Autodesk Inventor part; units mm, degrees
ref_plane "YZ Plane" through (0, 0, 0) normal (1, 0, 0) x (0, 1, 0)
ref_plane "XZ Plane" through (0, 0, 0) normal (0, 1, 0) x (-1, 0, 0)
ref_plane "XY Plane" through (0, 0, 0) normal (0, 0, 1) x (1, 0, 0)
sketch "草圖1" plane through (0, 0, 0) normal (0, 0, 1) x (1, 0, 0)
  line L0 (0, 0) -> (0, 10) construction
  line L1 (1.25, 0) -> (1.25, 10)
  line L2 (-1.25, 10) -> (-1.25, 0)
  arc A0 (-1.25, 0) -> (1.25, 0) centre (0, 0) ccw
  arc A1 (1.25, 10) -> (-1.25, 10) centre (0, 10) ccw
  circle A2 centre (0, 10) radius 0.625
  circle A3 centre (0, 0) radius 0.625
  point P0 (0, 5)
  dimension "d0" = 10
  dimension "d1" = 2.5
  dimension "d2" = 1.25
  dimension "d3" = 1.25
extrude "擠出1" add sketch "草圖1" along normal blind 2
properties part number "3"
Geometry check sheet. Reference: the model listing, model coordinates, mm. Give positions to 0.01 mm unless a question says otherwise; leave off trailing zeros. Loops run counter-clockwise (first coordinate to the right, second up) from the corner with the lowest first, then second, coordinate; pieces in that order, holes last. Notation, with made-up numbers: M -24.75,38.25 L 0.25,38.25 A16 ccw 0.25,68.25 Z; hole C -3,36 d1. An arc over 180 degrees is marked long. Answer as a JSON object with one key per item and string values. Group by question number.
Item 1: Gauge pin test, flat end, axial feed: pin 1 (0.8 mm diameter, centred on x = 0, y = 0, fed in from +Z). Record the tip position at first contact, or that the pin passes through.
Item 2: Sectioned sample at C-C on x = -0.75. Record the boundary of the cut face in (y, z).
Item 3: Sectioned sample at A-A on x = 0. Record the boundary of the cut face in (y, z) (3 decimals), plus the area to 3 significant figures.
Item 4: Sectioned sample at D-D on x = 0.5. Record the boundary of the cut face in (y, z) (3 decimals), plus the area to 3 significant figures.
Item 5: Material ranges on L1, parallel to Y at x = 0, z = 1 (3 decimals); L2, parallel to Y at x = 0.5, z = 0.6 (3 decimals); L3, parallel to X at y = -0.25, z = 0.15, recorded low to high.
Item 6: Sectioned sample at B-B on z = 1.4. Record the boundary of the cut face in (x, y) (3 decimals).
Item 7: Mould release check, pull along Y, two halves, no side actions. Record for faces 1 (the cylindrical face through (-0.03, 11.25, 0.99)), 2 (the flat face through (1.25, 5, 1)), 3 (the cylindrical face through (-0.14, 10.61, 0.99)): pulls with the +Y half, pulls with the -Y half, needs draft (parallel to the pull), parting line crosses it, or undercut.
Findings below:
{
 "1": {"pin 1": "through"},
 "2": {"outline": "M -1,0 L 11,0 L 11,2 L -1,2 Z"},
 "3": {"outline": "M -1.25,0 L -0.625,0 L -0.625,2 L -1.25,2 Z; M 0.625,0 L 9.375,0 L 9.375,2 L 0.625,2 Z; M 10.625,0 L 11.25,0 L 11.25,2 L 10.625,2 Z", "area": "20.0 mm2"},
 "4": {"outline": "M -1.146,0 L -0.375,0 L -0.375,2 L -1.146,2 Z; M 0.375,0 L 9.625,0 L 9.625,2 L 0.375,2 Z; M 10.375,0 L 11.146,0 L 11.146,2 L 10.375,2 Z", "area": "21.6 mm2"},
 "5": {"L1": "-1.25 to -0.625, 0.625 to 9.375, 10.625 to 11.25", "L2": "-1.146 to -0.375, 0.375 to 9.625, 10.375 to 11.146", "L3": "-1.22 to -0.57, 0.57 to 1.22"},
 "6": {"outline": "M -1.25,0 A1.25 ccw 1.25,0 L 1.25,10 A1.25 ccw -1.25,10 Z; hole C 0,0 d1.25; hole C 0,10 d1.25"},
 "7": {"face 1": "pulls with the +Y half", "face 2": "needs draft", "face 3": "undercut"}
}
